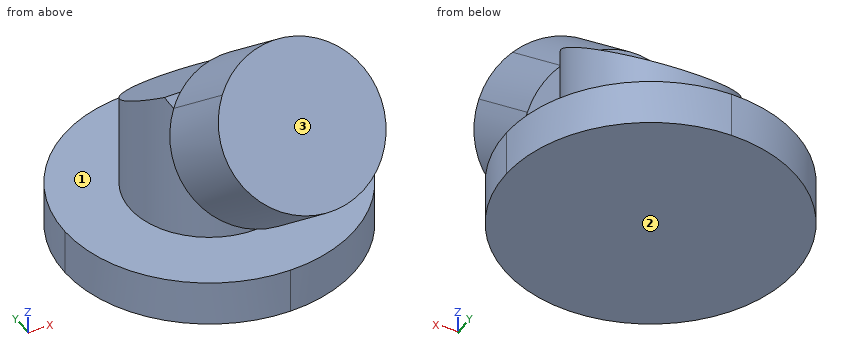
from build123d import *

# Parameters (mm, degrees)
F1_DEPTH = 32
F3_DEPTH = 50
F5_R     = 32
F5_R_2   = 17.5
F6_DEPTH = 40
F8_DEPTH = 25


with BuildPart() as f1:
    # F0 (on Right) → F1 (new body, symmetric)
    with BuildSketch(Plane.YZ):
        Polygon((-3.1593232416, 15), (32, 15), (-9.0026206753, 42.3286253849), (-31.9340601563, 15), align=None)
        Polygon((-32, 0), (32, 0), (32, 15), (-3.1593232416, 15), (-31.9340601563, 15), (-32, 15), align=None)
    extrude(amount=F1_DEPTH, both=True)

    # F2 (on face) → F3 (cut)
    with BuildSketch(Plane(origin=(0, 0, 0), x_dir=(1, 0, 0), z_dir=(0, 0, -1))):
        with BuildLine():
            ThreePointArc((-32, 0), (-22.6274170148, 22.6274169811), (-4.77e-08, 32))
            Line((-4.77e-08, 32), (-32, 32))
            Line((-32, 32), (-32, 0))
        make_face()
        with BuildLine():
            ThreePointArc((-4.77e-08, 32), (22.6274169811, 22.6274170148), (32, 0))
            Line((32, 0), (32, 32))
            Line((32, 32), (-4.77e-08, 32))
        make_face()
        with BuildLine():
            Line((32, -32), (32, 0))
            ThreePointArc((32, 0), (22.6274170148, -22.6274169811), (4.77e-08, -32))
            Line((4.77e-08, -32), (32, -32))
        make_face()
        with BuildLine():
            Line((-32, -32), (4.77e-08, -32))
            ThreePointArc((4.77e-08, -32), (-22.6274169811, -22.6274170148), (-32, 0))
            Line((-32, 0), (-32, -32))
        make_face()
    extrude(amount=-F3_DEPTH, mode=Mode.SUBTRACT)

    # F5 (on offset) → F6 (cut)
    with BuildSketch(Plane.XY.offset(50)):
        Circle(F5_R)
        Circle(F5_R_2, mode=Mode.SUBTRACT)
    extrude(amount=-F6_DEPTH, mode=Mode.SUBTRACT)

    # F7 (on face) → F8 (join)
    with BuildSketch(Plane(origin=(0, -26.1257339016, 21.9220936811), x_dir=(1, 0, 0), z_dir=(0, -0.7660444431, 0.6427876097))):
        with BuildLine():
            ThreePointArc((-13.8842207303, 24.0718845353), (-5.6247727608, -3.1521593573), (17.5, 13.4192597549))
            ThreePointArc((17.5, 13.4192597549), (16.5714191121, 19.0440325156), (13.8842207303, 24.0718845353))
            add(Edge.make_bspline(
                [(-13.8842207303, 24.0718845353), (0, -4.0807402451), (13.8842207303, 24.0718845353)],
                knots=[2.2441013689, 2.2441013689, 2.2441013689, 4.0390839383, 4.0390839383, 4.0390839383], degree=2, weights=[0.9413907542, 0.5730447129, 0.9413907542]))
        make_face()
        with BuildLine():
            add(Edge.make_bspline(
                [(-13.8842207303, 24.0718845353), (0, -4.0807402451), (13.8842207303, 24.0718845353)],
                knots=[2.2441013689, 2.2441013689, 2.2441013689, 4.0390839383, 4.0390839383, 4.0390839383], degree=2, weights=[0.9413907542, 0.5730447129, 0.9413907542]))
            ThreePointArc((13.8842207303, 24.0718845353), (12.7404400783, 25.4163921877), (11.4670320525, 26.6388352362))
            Line((11.4670320525, 26.6388352362), (-11.4670320525, 26.6388352362))
            ThreePointArc((-11.4670320525, 26.6388352362), (-12.7404400783, 25.4163921877), (-13.8842207303, 24.0718845353))
        make_face()
        with BuildLine():
            Line((-11.4670320525, 26.6388352362), (11.4670320525, 26.6388352362))
            ThreePointArc((11.4670320525, 26.6388352362), (0, 30.9192597549), (-11.4670320525, 26.6388352362))
        make_face()
    extrude(amount=F8_DEPTH)


solid = f1.part
Design review of the part built by this model. Coordinates are the model's own, in mm. Face numbers are marked on the shaded views. Round coordinates to 2 decimals unless told otherwise and drop trailing zeros. Loops run counter-clockwise (first coordinate to the right, second up) from the corner with the lowest first, then second, coordinate; pieces in that order, holes last. Notation, with made-up numbers: (26, -2) -> (41, -2) arc R27 ccw to (41, 37) -> close; hole circle Ø6 at (-6.75, 25). An arc over 180 degrees is marked (long way). Use one line per item in the form item = value. Start each with the question number.
Q1. For pin 1 Ø4 at (y, z) = (-19.5, 50) entering from +X; pin 2 Ø1.5 at (x, y) = (-8.5, -36.5) entering from +Z; pin 3 Ø12 at (x, y) = (12, -23.5) entering from -Z; pin 4 Ø1.5 at (y, z) = (-24, 45) entering from -X, all flat-tipped, find the tip position at first contact; note any pin that passes through.
Q2. Draft analysis for pull direction Z (two halves, no side actions). For the marked faces 1, 2 and 3, state which applies: +Z half, -Z half, draft (parallel to the pull), parting line (faces both ways), or undercut.
Q3. We need section A-A on x = -6.5. Give the boundary of the cut face in (y, z).
Q4. We need section C-C on z = 12.5. Give the boundary of the cut face in (x, y), then the cut area to 3 significant figures.
Q5. Wall thickness on line 1 along Z through (x, y) = (-19, 7.5); line 2 along Y through (x, z) = (-9, 14); line 3 along Y through (x, z) = (3.5, 32): over which ranges is each line inside the solid? List them lowest first. Write a range as [from, to].
Q6. We need section D-D on x = -26.5. Give the boundary of the cut face in (y, z).
Q7. We need section B-B on y = 7. Give the boundary of the cut face in (x, z).
Calculated:
q1.pin_1 = 14.11
q1.pin_2 = 49.35
q1.pin_3 = 0
q1.pin_4 = -16.81
q2.face_1 = undercut
q2.face_2 = -Z half
q2.face_3 = +Z half
q3.outline = (-47.1, 35.82) -> (-27.94, 19.76) -> (-16.25, 33.69) -> (-16.25, 10) -> (-31.33, 10) -> (-31.33, 0) -> (31.33, 0) -> (31.33, 10) -> (16.25, 10) -> (16.25, 25.5) -> (-9, 42.33) -> (-7.06, 44.65) -> (-26.21, 60.72) -> close
q4.outline = circle Ø35 at (0, 0)
q4.area = 962 mm²
q5.line_1 = [0, 10]
q5.line_2 = [-15.01, 15.01]
q5.line_3 = [-43.93, -17.67], [-17.15, 6.49]
q6.outline = (-17.94, 0) -> (17.94, 0) -> (17.94, 10) -> (-17.94, 10) -> close
q7.outline = (-31.22, 0) -> (31.22, 0) -> (31.22, 10) -> (16.04, 10) -> (16.04, 31.66) -> (-16.04, 31.66) -> (-16.04, 10) -> (-31.22, 10) -> close
